Design review of the part built by this model. Coordinates are the model's own, in mm. A direction names the side the tool comes from. Coordinates: 2 decimals unless noted, no trailing zeros. Write each loop counter-clockwise with the first axis right and the second up, starting at its lowest first coordinate (ties: lowest second). Pieces come first, ordered by that corner, then holes.
Q1. For L1, parallel to X at y = -52, z = -29; L2, parallel to Z at x = 4, y = -79.5; L3, parallel to Z at x = 28, y = -15.5, list the stretches that pass through material, from the lowest coordinate up.
Q2. Take a section at D-D, the plane x = 54. Write out the cut boundary in (y, z).
Q3. For pin 1 Ø15 at (x, z) = (36.19, 32.91) entering from +Y; pin 2 Ø13.5 at (x, z) = (9.5, 6) entering from +Y; pin 3 Ø2 at (x, y) = (49, -100.5) entering from -Z, all flat-tipped, find the tip position at first contact; note any pin that passes through.
Q4. Take a section at B-B, the plane y = -86.5. Write out the cut boundary in (x, z), plus the area to 3 significant figures.
Q5. Take a section at A-A, the plane y = -32.5. Write out the cut boundary in (x, z), plus the area to 3 significant figures.
Q6. The part is to be moulded in two halves that separate along Z. For faces 1 (the flat face through (36, -116.295, 33)), 2 (the flat face through (13, -39, -38.19)), 3 (the flat face through (-8, -91.295, -15)), say which applies: released by +Z, released by -Z, zero draft, split by the parting line, or undercut.
Q7. Take a section at C-C, the plane x = -4. Write out the cut boundary in (y, z).
Q8. For faces 4 (the flat face through (36, -116.295, -13)), 5 (the cylindrical face through (-2.474, -90.028, 19.874)), 6 (the cylindrical face through (-0.179, -103.62, 43.612)), list the 3-axis set-ups (+Z, -Z, +X, -X, +Y, -Y) from which the entire face can be reached by the end or side of a thin tool; tool diameter is ignored.
from build123d import *

# Parameters (mm, degrees)
F1_W      = 93.1631103158
F1_H      = 94.4140702486
F2_DEPTH  = 103.8612350821
F3_R      = 15
F4_DEPTH  = 25
F5_T      = -2.5
F6_DEPTH  = 25
F7_R      = 15.2680412387
F8_DEPTH  = 25
F9_R      = 13.6293819141
F10_DEPTH = 54.4321462512


with BuildPart() as f2:
    # F1 (on offset) → F2 (new body)
    with BuildSketch(Plane.XZ.offset(-12.5657636672)):
        with Locations((13.9752887189, 9.0170353651)):
            Rectangle(F1_W, F1_H)
    extrude(amount=F2_DEPTH)

    # F3 (on face) → F4 (join)
    with BuildSketch(Plane.XZ.offset(91.2954714149)):
        with Locations((36.1929880455, 32.9128091689)):
            Circle(F3_R)
        with Locations((36.1929880455, -12.9296954255)):
            Circle(F3_R)
        with Locations((-8.2424106076, -14.8787384387)):
            Circle(F3_R)
        with Locations((-8.2424106076, 30.9637661558)):
            Circle(F3_R)
    extrude(amount=F4_DEPTH)

    # F5
    f5_openings = [f2.faces().sort_by_distance(p)[0] for p in [
        (13.975289, 12.565764, 9.017035),
    ]]
    offset(amount=F5_T, openings=f5_openings, kind=Kind.INTERSECTION)

    # F3 (on face) → F6 (join)
    with BuildSketch(Plane.XZ.offset(91.2954714149)):
        with Locations((36.1929880455, 32.9128091689)):
            Circle(F3_R)
        with Locations((36.1929880455, -12.9296954255)):
            Circle(F3_R)
        with Locations((-8.2424106076, -14.8787384387)):
            Circle(F3_R)
        with Locations((-8.2424106076, 30.9637661558)):
            Circle(F3_R)
    extrude(amount=F6_DEPTH)

    # F7 (on face) → F8 (join)
    with BuildSketch(Plane.XZ.offset(91.2954714149)):
        with Locations((14.2471631989, 9.8856743425)):
            Circle(F7_R)
    extrude(amount=F8_DEPTH)

    # F9 (on face) → F10 (join)
    with BuildSketch(Plane.XZ.offset(91.2954714149)):
        with Locations((14.0535570681, 9.2893429101)):
            Circle(F9_R)
    extrude(amount=-F10_DEPTH)


solid = f2.part
Responses:
1. L1: x = -32.61 to -30.11, 58.06 to 60.56
1. L2: z = -38.19 to -35.69, 0.09 to 18.49, 53.72 to 56.22
1. L3: z = -38.19 to -35.69, 53.72 to 56.22
2. outline: (-91.3, -38.19) - (12.57, -38.19) - (12.57, -35.69) - (-88.8, -35.69) - (-88.8, 53.72) - (12.57, 53.72) - (12.57, 56.22) - (-91.3, 56.22) - close
3. pin 1: stops at y = -91.3
3. pin 2: stops at y = -36.86
3. pin 3: stops at z = -22.18
4. outline: (-32.61, -38.19) - (60.56, -38.19) - (60.56, 56.22) - (-32.61, 56.22) - close; circle Ø27.26 at (14.05, 9.29); hole (-30.11, -35.69) - (58.06, -35.69) - (58.06, 53.72) - (-30.11, 53.72) - close
4. area: 1,500 mm2
5. outline: (-32.61, -38.19) - (60.56, -38.19) - (60.56, 56.22) - (-32.61, 56.22) - close; hole (-30.11, -35.69) - (58.06, -35.69) - (58.06, 53.72) - (-30.11, 53.72) - close
5. area: 913 mm2
6. face 1: zero draft
6. face 2: released by -Z
6. face 3: undercut
7. outline: (-116.3, -29.27) - (-91.3, -29.27) - (-91.3, -38.19) - (12.57, -38.19) - (12.57, -35.69) - (-88.8, -35.69) - (-88.8, -26.64) - (-91.3, -26.64) - (-91.3, -3.12) - (-88.8, -3.12) - (-88.8, 19.21) - (-91.3, 19.21) - (-91.3, 42.72) - (-88.8, 42.72) - (-88.8, 53.72) - (12.57, 53.72) - (12.57, 56.22) - (-91.3, 56.22) - (-91.3, 45.35) - (-116.3, 45.35) - (-116.3, 16.58) - (-91.3, 16.58) - (-91.3, -0.49) - (-116.3, -0.49) - close
8. face 4: +Z, -Z, +X, -X, -Y
8. face 5: +Y
8. face 6: -Y
